```python
from build123d import *

# Parameters (mm, degrees)
CONG_1_R                = 2
ESQUISSE2_W             = 1.5
ESQUISSE2_H             = 6.244997998
ENL_V_MAT_EXTRU_1_DEPTH = 8
ESQUISSE3_R             = 1.5
ENL_V_MAT_EXTRU_2_DEPTH = 45.288824776


with BuildPart() as part:
    # Esquisse1 → Révolution1 (revolve)
    with BuildSketch(Plane.XY, mode=Mode.PRIVATE) as r_volution1_sk:
        Polygon((0, 0), (4, 0), (4, -26), (7.5, -26), (7.5, -43), (3, -43), (3, -29), (0, -26), align=None)
    revolve(r_volution1_sk.sketch.rotate(Axis((0, -26, 0), (0, -1, 0)), 180), axis=Axis((0, -26, 0), (0, -1, 0)))

    # Congé1
    cong_1_edges = [part.edges().sort_by_distance(p)[0] for p in [
        (4, -26, 0),
    ]]
    fillet(cong_1_edges, radius=CONG_1_R)

    # Esquisse2 → Enlèv. mat.-Extru.1 (cut)
    with BuildSketch(Plane(origin=(0, 0, 0), x_dir=(1, 0, 0), z_dir=(0, 1, 0))):
        with Locations((3.25, 0)):
            Rectangle(ESQUISSE2_W, ESQUISSE2_H)
    extrude(amount=-ENL_V_MAT_EXTRU_1_DEPTH, mode=Mode.SUBTRACT)

    # Esquisse3 → Enlèv. mat.-Extru.2 (cut, through all)
    with BuildSketch(Plane(origin=(0, 0, 0), x_dir=(0, 0, -1), z_dir=(1, 0, 0))):
        with Locations(Location((0, -34, 0), (0, 0, 180))):
            Circle(ESQUISSE3_R)
    extrude(amount=ENL_V_MAT_EXTRU_2_DEPTH, mode=Mode.SUBTRACT)


solid = part.part
```
Geometry: final body of the model. Coordinates: model frame, mm. A direction names the side the tool comes from. Round coordinates to 2 decimals unless told otherwise and drop trailing zeros. Order: outer loops, then holes, each group sorted by start corner. A loop starts at its lowest first (then second) coordinate and runs counter-clockwise, first axis right, second up. Notation, with made-up numbers: M -38,6 L 20,6 A23 cw 20,15 Z; hole C 79.25,69 d5. An arc over 180 degrees is marked long. Use one line per item in the form item = value. Start each with the question number.
Q1. Access query for faces 4 (the face through (3, -8, 0)), 5 (the face through (-2.86, -35.9, -0.9)), 6 (the face through (-1, 0, 0)). Directions: +Z, -Z, +X, -X, +Y, -Y. A direction counts if a zero-diameter tool reaches every point of the face in a straight line with its end or side. Return the directions, or none.
Q2. Material intervals for line 1 (Z direction, x = 0, y = -34); line 2 (X direction, y = -32, z = -1.5); line 3 (Y direction, x = 6.75, z = 1), sorted ascending. Write a range as [from, to].
Q3. Cut plane A-A (y = -36). Return loops of the section in (x, z), and give its area (3 significant figures).
Q4. Pin query (flat end, axial travel): pin 1 Ø1.5 at (y, z) = (-33.5, -5.5) entering from +X; pin 2 Ø2 at (x, y) = (3, -8) entering from +Z; pin 3 Ø1.6 at (x, z) = (3.5, -1.5) entering from +Y. Return the tip coordinate at first contact, or that it passes through.
Q5. Mould query, pull axis Z, two halves, no side actions, for faces 1 (the face through (5.02, -34.07, -1.5)), 2 (the face through (-3.695, -12.168, 1.532)), 3 (the face through (2, -26, -6)). Classes: +Z half, -Z half, draft (parallel to the pull), parting line (faces both ways), or undercut.
Q6. Cut plane B-B (y = -16). Return loops of the section in (x, z).
Geometry results:
q1.face_4 = +Z, -Z, +X, +Y
q1.face_5 = -Y
q1.face_6 = +Z, -Z, +X, -X, +Y
q2.line_1 = [-7.5, -3], [3, 7.5]
q2.line_2 = [-7.35, -2.6], [2.6, 7.35]
q2.line_3 = [-43, -35.12], [-32.88, -26]
q3.outline = C 0,0 d15; hole C 0,0 d6
q3.area = 148 mm^2
q4.pin_1 = 5.8
q4.pin_2 = 3.46
q4.pin_3 = -8
q5.face_1 = undercut
q5.face_2 = parting line
q5.face_3 = draft
q6.outline = C 0,0 d8
